from build123d import *

# Parameters (mm, degrees)
SKETCH1_W           = 170
SKETCH1_H           = 40
SKETCH1_R           = 2.5
BOSS_EXTRUDE1_DEPTH = 10
SKETCH2_W           = 10
SKETCH2_H           = 40
BOSS_EXTRUDE2_DEPTH = 70
SKETCH3_W           = 20
SKETCH3_H           = 40
CUT_EXTRUDE1_DEPTH  = 50
SKETCH4_R           = 2.5
CUT_EXTRUDE2_DEPTH  = 24


with BuildPart() as part:
    # Sketch1 → Boss-Extrude1 (new body)
    with BuildSketch(Plane(origin=(0, 0, 0), x_dir=(1, 0, 0), z_dir=(0, 1, 0))):
        Rectangle(SKETCH1_W, SKETCH1_H)
        with Locations(Location((0, 0, 0), (0, 0, 270))):
            Circle(SKETCH1_R, mode=Mode.SUBTRACT)
    extrude(amount=BOSS_EXTRUDE1_DEPTH)

    # Sketch2 → Boss-Extrude2 (add)
    with BuildSketch(Plane(origin=(0, 10, 0), x_dir=(1, 0, 0), z_dir=(0, 1, 0))):
        with Locations((80, 0)):
            Rectangle(SKETCH2_W, SKETCH2_H)
        with Locations((-80, 0)):
            Rectangle(SKETCH2_W, SKETCH2_H)
    extrude(amount=BOSS_EXTRUDE2_DEPTH)

    # Sketch3 → Cut-Extrude1 (cut)
    with BuildSketch(Plane.ZY.offset(85)):
        with Locations((0, 50)):
            Rectangle(SKETCH3_W, SKETCH3_H)
        with BuildLine():
            Line((3, 80), (3, 76.5))
            ThreePointArc((3, 76.5), (0, 73.5), (-3, 76.5))
            Line((-3, 76.5), (-3, 80))
            ThreePointArc((-3, 80), (0, 83), (3, 80))
        make_face()
    extrude(amount=-CUT_EXTRUDE1_DEPTH, mode=Mode.SUBTRACT)

    # Sketch4 → Cut-Extrude2 (cut)
    with BuildSketch(Plane(origin=(85, 0, 0), x_dir=(0, 0, -1), z_dir=(1, 0, 0))):
        with Locations((0, 60)):
            Circle(SKETCH4_R)
    extrude(amount=-CUT_EXTRUDE2_DEPTH, mode=Mode.SUBTRACT)


solid = part.part
For this review, take the finished solid that the model builds, in its own axes (mm). A direction names the side the tool comes from. Round coordinates to 2 decimals unless told otherwise and drop trailing zeros. Write each loop counter-clockwise with the first axis right and the second up, starting at its lowest first coordinate (ties: lowest second). Pieces come first, ordered by that corner, then holes. Notation, with made-up numbers: (83.5, 85.5) -> (104.5, 85.5) arc R18 ccw to (104.5, 120.5) -> close; hole circle Ø4 at (38, 2.5). An arc over 180 degrees is marked (long way). Put each result on its own line as item: value.
Q1. Consider section C-C on y = 43. State the section outline as (x, z) points, and give its area (3 significant figures).
Determined:
outline: (-85, -20) -> (-75, -20) -> (-75, -10) -> (-85, -10) -> close; (-85, 10) -> (-75, 10) -> (-75, 20) -> (-85, 20) -> close; (75, -20) -> (85, -20) -> (85, 20) -> (75, 20) -> close
area: 600 mm^2
Q2. To check wall thickness, follow L1, parallel to X at y = 25, z = -17.5; L2, parallel to Y at x = 81, z = 0; L3, parallel to X at y = 6, z = 0. State the ranges of each line that lie inside material, in increasing order. Write a range as [from, to].
Determined:
L1: x = [-85, -75], [75, 85]
L2: y = [0, 57.5], [62.5, 80]
L3: x = [-85, -2.5], [2.5, 85]
Q3. Consider section B-B on z = 8. State the section outline as (x, y) points.
Determined:
outline: (-85, 0) -> (85, 0) -> (85, 80) -> (75, 80) -> (75, 10) -> (-75, 10) -> (-75, 30) -> (-85, 30) -> close; (-85, 70) -> (-75, 70) -> (-75, 80) -> (-85, 80) -> close
Q4. Consider section D-D on z = 0. State the section outline as (x, y) points.
Determined:
outline: (-85, 0) -> (-2.5, 0) -> (-2.5, 10) -> (-75, 10) -> (-75, 30) -> (-85, 30) -> close; (-85, 70) -> (-75, 70) -> (-75, 73.5) -> (-85, 73.5) -> close; (2.5, 0) -> (85, 0) -> (85, 57.5) -> (75, 57.5) -> (75, 10) -> (2.5, 10) -> close; (75, 62.5) -> (85, 62.5) -> (85, 80) -> (75, 80) -> close
Q5. The part is to be moulded in two halves that separate along X. For faces 1 (the flat face through (-85, 22, 0)), 2 (the flat face through (-80, 70, 0)), 3 (the flat face through (-75, 29, 0)), say which applies: released by +X, released by -X, zero draft, split by the parting line, or undercut.
Determined:
face 1: released by -X
face 2: zero draft
face 3: undercut
Q6. Machinability: for faces 4 (the flat face through (-1, 10, -5)), 5 (the flat face through (-80, 78, 3)), 6 (the cylindrical face through (80.07, 57.56, 0.54)), 7 (the flat face through (-80, 30, 0)), 8 (the flat face through (80, 80, 0)), which of the approach directions +Z, -Z, +X, -X, +Y, -Y give a long, thin tool a straight path to every point of the face, cutting with its end or side? Answer none if there is none.
Determined:
face 4: +Z, -Z, +Y
face 5: -X, +Y
face 6: +X, -X
face 7: -X
face 8: +Z, -Z, +X, -X, +Y
Q7. Consider section A-A on y = 25. State the section outline as (x, z) points, and give its area (3 significant figures).
Determined:
outline: (-85, -20) -> (-75, -20) -> (-75, 20) -> (-85, 20) -> close; (75, -20) -> (85, -20) -> (85, 20) -> (75, 20) -> close
area: 800 mm^2
Q8. Clearance check with a flat-ended pin moving along its axis: pin 1 Ø20 at (x, z) = (9, -8.5) entering from +Y. State where the tip first meets the part, or that it passes through.
Determined:
pin 1: stops at y = 10
